Check sheet for the modelled part. Datum: model origin and axes. Units: mm. A direction names the side the tool comes from. Give positions to 0.01 mm unless a question says otherwise; leave off trailing zeros. Order: outer loops, then holes, each group sorted by start corner. A loop starts at its lowest first (then second) coordinate and runs counter-clockwise, first axis right, second up.
Item 1: Sectioned sample at D-D on x = 8.5. Record the boundary of the cut face in (y, z) (3 decimals).
Item 2: Sectioned sample at A-A on x = 14. Record the boundary of the cut face in (y, z) (3 decimals).
Item 3: Sectioned sample at C-C on y = 24.75. Record the boundary of the cut face in (x, z).
Item 4: Gauge pin test, flat ends, axial feed: P1, Ø8, axis at y = 14, z = 14, coming from the +X side; P2, Ø1.8, axis at y = 14, z = 13, coming from the +X side; P3, Ø2.5, axis at x = 14, z = 3.5, coming from the +Y side; P4, Ø1.9, axis at x = 14.5, y = 15, coming from the -Z side. Record the tip position at first contact, or that the pin passes through.
Item 5: Access from +Z, -Z, +X, -X, +Y, -Y to the whole of each face (thin tool, end or side, straight path). Record for faces 1 (the cylindrical face through (23.1, 12.2, 16.4)), 2 (the flat face through (10, 14, 14)), 3 (the cylindrical face through (11.6, 12.2, 23.1)), 4 (the cylindrical face through (12.5, 11.2, 4.9)), 5 (the cylindrical face through (4.886, 22.478, 14.575)).
Item 6: Material ranges on line 1 along X through (y, z) = (20.5, 3.5); line 2 along Y through (x, z) = (14, 22); line 3 along X through (y, z) = (25.5, 13.25), recorded low to high.
Item 7: Release check for a two-part mould opening along X. For faces 6 (the flat face through (14, 0, 14)), 7 (the flat face through (18, 14, 14)), 8 (the flat face through (14, 14, 18)) record: released by +X, released by -X, zero draft, split by the parting line, or undercut.
Item 8: Sectioned sample at B-B on z = 3.5. Record the boundary of the cut face in (x, y) (3 decimals), and give its area (3 significant figures).
from build123d import *

# Parameters (mm, degrees)
CROQUIS1_W              = 28
CROQUIS1_H              = 28
SALIENTE_EXTRUIR1_DEPTH = 28
CROQUIS4_R              = 3.175
CORTAR_EXTRUIR3_DEPTH   = 10
CROQUIS6_R              = 3
CORTAR_EXTRUIR4_DEPTH   = 10
CROQUIS8_R              = 3.175
CORTAR_EXTRUIR5_DEPTH   = 10
CROQUIS9_R              = 3
CORTAR_EXTRUIR6_DEPTH   = 10
CROQUIS10_R             = 1.5
CORTAR_EXTRUIR7_DEPTH   = 12


with BuildPart() as part:
    # Croquis1 → Saliente-Extruir1 (new body)
    with BuildSketch(Plane.XY):
        with Locations((14, 14)):
            Rectangle(CROQUIS1_W, CROQUIS1_H)
    extrude(amount=SALIENTE_EXTRUIR1_DEPTH)

    # Croquis4 → Cortar-Extruir3 (cut)
    with BuildSketch(Plane.ZY):
        with Locations((14, 14)):
            Circle(CROQUIS4_R)
    extrude(amount=-CORTAR_EXTRUIR3_DEPTH, mode=Mode.SUBTRACT)

    # Croquis6 → Cortar-Extruir4 (cut)
    with BuildSketch(Plane(origin=(28, 0, 0), x_dir=(0, 0, -1), z_dir=(1, 0, 0))):
        with Locations((-14, 14)):
            Circle(CROQUIS6_R)
    extrude(amount=-CORTAR_EXTRUIR4_DEPTH, mode=Mode.SUBTRACT)

    # Croquis8 → Cortar-Extruir5 (cut)
    with BuildSketch(Plane(origin=(0, 0, 0), x_dir=(-1, 0, 0), z_dir=(0, 0, -1))):
        with Locations((-14, 14)):
            Circle(CROQUIS8_R)
    extrude(amount=-CORTAR_EXTRUIR5_DEPTH, mode=Mode.SUBTRACT)

    # Croquis9 → Cortar-Extruir6 (cut)
    with BuildSketch(Plane.XY.offset(28)):
        with Locations((14, 14)):
            Circle(CROQUIS9_R)
    extrude(amount=-CORTAR_EXTRUIR6_DEPTH, mode=Mode.SUBTRACT)

    # Croquis10 → Cortar-Extruir7 (cut)
    with BuildSketch(Plane(origin=(0, 28, 0), x_dir=(1, 0, 0), z_dir=(0, 1, 0))):
        with Locations((3.5, -14)):
            Circle(CROQUIS10_R)
        with Locations((14, -3.5)):
            Circle(CROQUIS10_R)
    extrude(amount=-CORTAR_EXTRUIR7_DEPTH, mode=Mode.SUBTRACT)


solid = part.part
Report:
1. outline: (0, 0) - (28, 0) - (28, 28) - (0, 28) - close; hole circle Ø6.35 at (14, 14)
2. outline: (0, 0) - (10.825, 0) - (10.825, 10) - (17.175, 10) - (17.175, 5) - (28, 5) - (28, 28) - (17, 28) - (17, 18) - (11, 18) - (11, 28) - (0, 28) - close; (17.175, 0) - (28, 0) - (28, 2) - (17.175, 2) - close
3. outline: (0, 0) - (28, 0) - (28, 28) - (0, 28) - close; hole circle Ø3 at (3.5, 14); hole circle Ø3 at (14, 3.5)
4. P1: stops at x = 28
4. P2: stops at x = 18
4. P3: stops at y = 11.08
4. P4: stops at z = 10
5. face 1: +X
5. face 2: -X
5. face 3: +Z
5. face 4: -Z
5. face 5: +Y
6. line 1: x = 0 to 12.5, 15.5 to 28
6. line 2: y = 0 to 11, 17 to 28
6. line 3: x = 0 to 2.2, 4.8 to 28
7. face 6: zero draft
7. face 7: released by +X
7. face 8: undercut
8. outline: (0, 0) - (28, 0) - (28, 28) - (15.5, 28) - (15.5, 16.798) arc R3.175 cw (long way) to (12.5, 16.798) - (12.5, 28) - (0, 28) - close
8. area: 719 mm2
